```python
from build123d import *

# Parameters (mm, degrees)
SKETCH_1_W          = 225
SKETCH_1_H          = 162
EXTRUDE_1_DEPTH     = 5
SKETCH_3_W          = 212
SKETCH_3_H          = 150
EXTRUDE_2_DEPTH     = 19
EXTRUDE_3_DEPTH     = 10
SKETCH_5_W          = 20
SKETCH_5_H          = 65.649810637
SKETCH_5_H_2        = 64
CUT_EXTRUDE_1_DEPTH = 10
SKETCH_7_R          = 2
SKETCH_7_W          = 8
SKETCH_7_H          = 12
SKETCH_7_R_2        = 0.262594618
SKETCH_7_R_3        = 0.290999542
EXTRUDE_4_DEPTH     = 5


with BuildPart() as part:
    # 草图1 → 凸台-拉伸1 (new body)
    with BuildSketch(Plane.XY):
        with Locations((112.5, 81)):
            Rectangle(SKETCH_1_W, SKETCH_1_H)
    extrude(amount=EXTRUDE_1_DEPTH)

    # 草图3 → 凸台-拉伸2 (add)
    with BuildSketch(Plane(origin=(0, 0, 0), x_dir=(-1, 0, 0), z_dir=(0, 0, -1))):
        with Locations((-112.5, 81)):
            Rectangle(SKETCH_3_W, SKETCH_3_H)
    extrude(amount=EXTRUDE_2_DEPTH)

    # 草图4 → 凸台-拉伸3 (add)
    with BuildSketch(Plane(origin=(0, 0, -19), x_dir=(-1, 0, 0), z_dir=(0, 0, -1))):
        Polygon((-112.5, 136), (-188, 136), (-188, 26), (-37, 26), (-37, 136), align=None)
    extrude(amount=EXTRUDE_3_DEPTH)

    # 草图5 → 切除-拉伸1 (cut)
    with BuildSketch(Plane(origin=(0, 0, -29), x_dir=(-1, 0, 0), z_dir=(0, 0, -1))):
        with Locations((-178, 88.175094682)):
            Rectangle(SKETCH_5_W, SKETCH_5_H)
        with Locations((-47, 89)):
            Rectangle(SKETCH_5_W, SKETCH_5_H_2)
    extrude(amount=-CUT_EXTRUDE_1_DEPTH, mode=Mode.SUBTRACT)

    # 草图7 → 凸台-拉伸4 (add)
    with BuildSketch(Plane(origin=(0, 0, -19), x_dir=(-1, 0, 0), z_dir=(0, 0, -1))):
        with Locations((-50, 65.359909726)):
            Circle(SKETCH_7_R)
        with Locations((-50, 91.297088519)):
            Circle(SKETCH_7_R)
        with Locations((-50, 111.883776524)):
            Rectangle(SKETCH_7_W, SKETCH_7_H)
        with Locations((-50, 115.545534251)):
            Circle(SKETCH_7_R_2, mode=Mode.SUBTRACT)
        with Locations((-50, 108.299645663)):
            Circle(SKETCH_7_R_3, mode=Mode.SUBTRACT)
        with BuildLine():
            Line((-54, 84.588527339), (-54, 72.068223644))
            ThreePointArc((-54, 72.068223644), (-52.877182181, 69.728098207), (-50.349208627, 69.139662463))
            Line((-50.349208627, 69.139662463), (-47.349208627, 69.80632913))
            ThreePointArc((-47.349208627, 69.80632913), (-45.659874563, 70.85770813), (-45, 72.73489031))
            Line((-45, 72.73489031), (-45, 83.921860672))
            ThreePointArc((-45, 83.921860672), (-45.659874563, 85.799042853), (-47.349208627, 86.850421853))
            Line((-47.349208627, 86.850421853), (-50.349208627, 87.517088519))
            ThreePointArc((-50.349208627, 87.517088519), (-52.877182181, 86.928652776), (-54, 84.588527339))
        make_face()
    extrude(amount=EXTRUDE_4_DEPTH)


solid = part.part
```
Source: CAD feature listing. Evaluate the final solid. Frame: model axes, mm. A direction names the side the tool comes from. Coordinates: 2 decimals unless noted, no trailing zeros. Order: outer loops, then holes, each group sorted by start corner. A loop starts at its lowest first (then second) coordinate and runs counter-clockwise, first axis right, second up. Notation, with made-up numbers: M 57.5,42 L 83.5,42 A32 ccw 83.5,74 Z; hole C 29,27.25 d10. An arc over 180 degrees is marked long. Write each question's results on one line, items separated by ' | '. Start each with the question number.
1) Section query C-C (y = 78). Return the cut outline in (x, z), plus the area to 3 significant figures.
2) Contact query for flat-ended pins moving along their axis: pin 1 Ø11 at (y, z) = (39, -22) entering from +X; pin 2 Ø9 at (x, y) = (48.5, 111.5) entering from -Z; pin 3 Ø5.5 at (x, z) = (49.5, -22) entering from -Y. Output: stop coordinate, or through.
3) Section query A-A (y = 37). Return the cut outline in (x, z).
4) Line query: line 1 (Y direction, x = 132, z = -25); line 2 (Z direction, x = 36, y = 133.5); line 3 (X direction, y = 7, z = -8). Output: solid intervals per line, ascending. Write a range as from..to.
5) Access query for faces 4 (the face through (50, 112, -24)), 5 (the face through (178, 121, -24)), 6 (the face through (37, 41, -24)). Directions: +Z, -Z, +X, -X, +Y, -Y. A direction counts if a zero-diameter tool reaches every point of the face in a straight line with its end or side. Return the directions, or none.
6) Draft query along X for faces 1 (the face through (54, 78, -21)), 2 (the face through (0, 80, 2)), 3 (the face through (50, 117.884, -21)). Return one class per face: released by +X, released by -X, zero draft, split by the parting line, or undercut.
7) Section query D-D (z = -12.5). Return the cut outline in (x, y), plus the area to 3 significant figures.
8) Section query B-B (x = 78.5). Return the cut outline in (y, z), plus the area to 3 significant figures.
Answers:
1) outline: M 0,0 L 6.5,0 L 6.5,-19 L 45,-19 L 45,-24 L 54,-24 L 54,-19 L 57,-19 L 57,-29 L 168,-29 L 168,-19 L 218.5,-19 L 218.5,0 L 225,0 L 225,5 L 0,5 Z | area: 6,310 mm^2
2) pin 1: stops at x = 218.5 | pin 2: stops at z = -24 | pin 3: stops at y = 26
3) outline: M 0,0 L 6.5,0 L 6.5,-19 L 37,-19 L 37,-29 L 188,-29 L 188,-19 L 218.5,-19 L 218.5,0 L 225,0 L 225,5 L 0,5 Z
4) line 1: y = 26..136 | line 2: z = -19..5 | line 3: x = 6.5..218.5
5) face 4: -Z, -X | face 5: -Z, +X | face 6: -Z, -X, +Y, -Y
6) face 1: undercut | face 2: released by -X | face 3: zero draft
7) outline: M 6.5,6 L 218.5,6 L 218.5,156 L 6.5,156 Z | area: 31,800 mm^2
8) outline: M 0,0 L 6,0 L 6,-19 L 26,-19 L 26,-29 L 136,-29 L 136,-19 L 156,-19 L 156,0 L 162,0 L 162,5 L 0,5 Z | area: 4,760 mm^2
